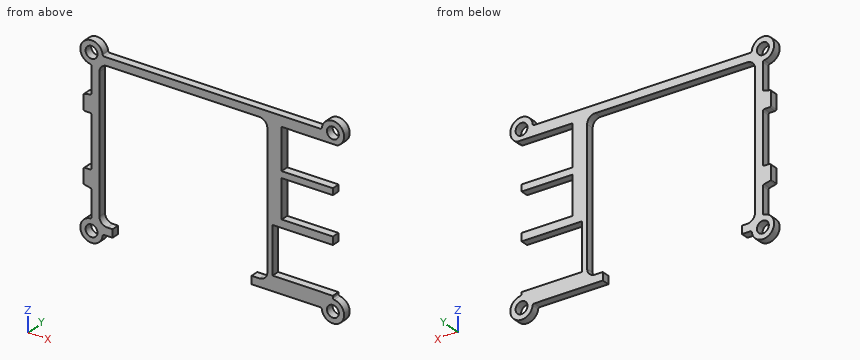
from build123d import *

# Parameters (mm, degrees)
SKETCH1_R           = 2.265
BOSS_EXTRUDE1_DEPTH = 3
SKETCH2_W           = 6.5
SKETCH2_H           = 20
CUT_EXTRUDE1_DEPTH  = 3
BOSS_EXTRUDE2_DEPTH = 3
CUT_EXTRUDE2_DEPTH  = 3
SKETCH5_W           = 3
SKETCH5_H           = 20
BOSS_EXTRUDE3_DEPTH = 3
SKETCH6_W           = 27.010134686
SKETCH6_H           = 17.9
CUT_EXTRUDE3_DEPTH  = 3
SKETCH7_W           = 19.5
SKETCH7_H           = 14.6
CUT_EXTRUDE4_DEPTH  = 3
SKETCH8_W           = 19.5
SKETCH8_H           = 15.6
CUT_EXTRUDE5_DEPTH  = 3
SKETCH9_W           = 2.019620965
SKETCH9_H           = 0.574286347
CUT_EXTRUDE6_DEPTH  = 3
FILLET1_R           = 0.6
SKETCH10_W          = 53
SKETCH10_H          = 3
CUT_EXTRUDE7_DEPTH  = 10


with BuildPart() as part:
    # Sketch1 → Boss-Extrude1 (new body)
    with BuildSketch(Plane(origin=(0, 0, 0), x_dir=(1, 0, 0), z_dir=(0, 1, 0))):
        with BuildLine():
            Line((4.265, 0), (87.735, 0))
            ThreePointArc((87.735, 0), (95.015810422, 3.015810422), (92, -4.265))
            Line((92, -4.265), (92, -58.735))
            ThreePointArc((92, -58.735), (95.015810422, -66.015810422), (87.735, -63))
            Line((87.735, -63), (4.265, -63))
            ThreePointArc((4.265, -63), (-3.015810422, -66.015810422), (0, -58.735))
            Line((0, -58.735), (0, -4.265))
            ThreePointArc((0, -4.265), (-3.015810422, 3.015810422), (4.265, 0))
        make_face()
        with Locations(Location((0, 0, 0), (0, 0, 270))):
            Circle(SKETCH1_R, mode=Mode.SUBTRACT)
        with Locations(Location((92, 0, 0), (0, 0, 270))):
            Circle(SKETCH1_R, mode=Mode.SUBTRACT)
        with Locations(Location((92, -63, 0), (0, 0, 270))):
            Circle(SKETCH1_R, mode=Mode.SUBTRACT)
        with Locations(Location((0, -63, 0), (0, 0, 270))):
            Circle(SKETCH1_R, mode=Mode.SUBTRACT)
    extrude(amount=BOSS_EXTRUDE1_DEPTH)

    # Sketch2 → Cut-Extrude1 (cut)
    with BuildSketch(Plane(origin=(0, 3, 0), x_dir=(1, 0, 0), z_dir=(0, 1, 0))):
        with Locations((3.25, -31.5)):
            Rectangle(SKETCH2_W, SKETCH2_H)
    extrude(amount=-CUT_EXTRUDE1_DEPTH, mode=Mode.SUBTRACT)

    # Sketch3 → Boss-Extrude2 (add)
    with BuildSketch(Plane(origin=(0, 3, 0), x_dir=(1, 0, 0), z_dir=(0, 1, 0))):
        with BuildLine():
            Line((-2.7, -15.5), (0, -14.9))
            Line((0, -14.9), (0, -21.5))
            Line((0, -21.5), (-2.5, -21.5))
            ThreePointArc((-2.5, -21.5), (-2.853553391, -21.353553391), (-3, -21))
            Line((-3, -21), (-3, -15.8))
            ThreePointArc((-3, -15.8), (-2.912132034, -15.587867966), (-2.7, -15.5))
        make_face()
        with BuildLine():
            Line((-3, -42), (-3, -47.2))
            ThreePointArc((-3, -47.2), (-2.912132034, -47.412132034), (-2.7, -47.5))
            Line((-2.7, -47.5), (0, -48.1))
            Line((0, -48.1), (0, -41.5))
            Line((0, -41.5), (-2.5, -41.5))
            ThreePointArc((-2.5, -41.5), (-2.853553391, -41.646446609), (-3, -42))
        make_face()
    extrude(amount=-BOSS_EXTRUDE2_DEPTH)

    # Sketch4 → Cut-Extrude2 (cut)
    with BuildSketch(Plane(origin=(0, 3, 0), x_dir=(1, 0, 0), z_dir=(0, 1, 0))):
        with BuildLine():
            Line((6, -3), (64, -3))
            ThreePointArc((64, -3), (66.121320344, -3.878679656), (67, -6))
            Line((67, -6), (67, -57))
            ThreePointArc((67, -57), (66.121320344, -59.121320344), (64, -60))
            Line((64, -60), (6, -60))
            ThreePointArc((6, -60), (3.878679656, -59.121320344), (3, -57))
            Line((3, -57), (3, -6))
            ThreePointArc((3, -6), (3.878679656, -3.878679656), (6, -3))
        make_face()
    extrude(amount=-CUT_EXTRUDE2_DEPTH, mode=Mode.SUBTRACT)

    # Sketch5 → Boss-Extrude3 (add)
    with BuildSketch(Plane(origin=(0, 3, 0), x_dir=(1, 0, 0), z_dir=(0, 1, 0))):
        with Locations((1.5, -31.5)):
            Rectangle(SKETCH5_W, SKETCH5_H)
    extrude(amount=-BOSS_EXTRUDE3_DEPTH)

    # Sketch6 → Cut-Extrude3 (cut)
    with BuildSketch(Plane(origin=(0, 3, 0), x_dir=(1, 0, 0), z_dir=(0, 1, 0))):
        with Locations((82.505067343, -14.45)):
            Rectangle(SKETCH6_W, SKETCH6_H)
    extrude(amount=-CUT_EXTRUDE3_DEPTH, mode=Mode.SUBTRACT)

    # Sketch7 → Cut-Extrude4 (cut)
    with BuildSketch(Plane(origin=(0, 3, 0), x_dir=(1, 0, 0), z_dir=(0, 1, 0))):
        with Locations((82.25, -33.7)):
            Rectangle(SKETCH7_W, SKETCH7_H)
    extrude(amount=-CUT_EXTRUDE4_DEPTH, mode=Mode.SUBTRACT)

    # Sketch8 → Cut-Extrude5 (cut)
    with BuildSketch(Plane(origin=(0, 3, 0), x_dir=(1, 0, 0), z_dir=(0, 1, 0))):
        with Locations((82.25, -51.3)):
            Rectangle(SKETCH8_W, SKETCH8_H)
    extrude(amount=-CUT_EXTRUDE5_DEPTH, mode=Mode.SUBTRACT)

    # Sketch9 → Cut-Extrude6 (cut)
    with BuildSketch(Plane(origin=(0, 3, 0), x_dir=(1, 0, 0), z_dir=(0, 1, 0))):
        with Locations((93.009810483, -58.812856827)):
            Rectangle(SKETCH9_W, SKETCH9_H)
    extrude(amount=-CUT_EXTRUDE6_DEPTH, mode=Mode.SUBTRACT)

    # Fillet1
    fillet1_edges = [part.edges().sort_by_distance(p)[0] for p in [
        (0, 1.5, 41.5),
        (92, 1.5, 4.265),
        (0, 1.5, 21.5),
        (87.735, 1.5, 63),
        (4.265, 1.5, 63),
        (0, 1.5, 58.735),
        (0, 1.5, 4.265),
        (4.265, 1.5, 0),
        (87.735, 1.5, 0),
        (93.726332818, 1.5, 59.1),
        (0, 1.5, 14.9),
        (0, 1.5, 48.1),
    ]]
    fillet(fillet1_edges, radius=FILLET1_R)

    # Sketch10 → Cut-Extrude7 (cut)
    with BuildSketch(Plane(origin=(0, 3, 0), x_dir=(1, 0, 0), z_dir=(0, 1, 0))):
        with Locations((34.5, -1.5)):
            Rectangle(SKETCH10_W, SKETCH10_H)
    extrude(amount=-CUT_EXTRUDE7_DEPTH, mode=Mode.SUBTRACT)


solid = part.part
Source: CAD feature listing. Evaluate the final solid. Frame: model axes, mm. Round coordinates to 2 decimals unless told otherwise and drop trailing zeros. Loops run counter-clockwise (first coordinate to the right, second up) from the corner with the lowest first, then second, coordinate; pieces in that order, holes last. Notation, with made-up numbers: (-35.5, -7) -> (-6.5, -7) arc R24 ccw to (-6.5, 29) -> close; hole circle Ø4 at (-17.75, 28.25). An arc over 180 degrees is marked (long way). Answer as a JSON object with one key per item and string values. Group by question number.
Q1. Section query A-A (z = 33). Output: boundary loops of the cut face in (x, y), plus the area to 3 significant figures.
Q2. Ray query, line 1 (Z direction, x = 85, y = 1.55); line 2 (X direction, y = 1.2, z = 39); line 3 (X direction, y = 1.9, z = 23.5). Return the intervals inside material, ascending. Write a range as from..to.
Q3. Section query B-B (x = 62). Output: boundary loops of the cut face in (y, z).
Q4. Section query C-C (x = 74). Output: boundary loops of the cut face in (y, z), plus the area to 3 significant figures.
Q5. Section query D-D (x = 50.5). Output: boundary loops of the cut face in (y, z).
Q6. Contact query for flat-ended pins moving along their axis: P1, Ø1.5, axis at y = 2, z = 30, coming from the +X side; P2, Ø5, axis at x = 84.5, z = 45.5, coming from the +Y side; P3, Ø1, axis at x = 50, y = 1.5, coming from the +Z side; P4, Ø1.5, axis at x = 80, y = 1.5, coming from the -Z side. Output: stop coordinate, or through.
Completed:
{
 "1": {"outline": "(0, 0) -> (3, 0) -> (3, 3) -> (0, 3) -> close; (67, 0) -> (72.5, 0) -> (72.5, 3) -> (67, 3) -> close", "area": "25.5 mm²"},
 "2": {"line 1": "0..5.5, 23.4..26.4, 41..43.5, 59.1..63", "line 2": "0..3, 67..72.5", "line 3": "0..3, 67..92"},
 "3": {"outline": "(0, 0) -> (3, 0) -> (3, 3) -> (0, 3) -> close; (0, 60) -> (3, 60) -> (3, 63) -> (0, 63) -> close"},
 "4": {"outline": "(0, 0) -> (3, 0) -> (3, 5.5) -> (0, 5.5) -> close; (0, 23.4) -> (3, 23.4) -> (3, 26.4) -> (0, 26.4) -> close; (0, 41) -> (3, 41) -> (3, 43.5) -> (0, 43.5) -> close; (0, 59.1) -> (3, 59.1) -> (3, 63) -> (0, 63) -> close", "area": "44.7 mm²"},
 "5": {"outline": "(0, 60) -> (3, 60) -> (3, 63) -> (0, 63) -> close"},
 "6": {"P1": "x = 72.5", "P2": "y = 3", "P3": "z = 63", "P4": "z = 0"}
}
